Check sheet for the modelled part. Datum: model origin and axes. Units: mm. Coordinates: 2 decimals unless noted, no trailing zeros. Order: outer loops, then holes, each group sorted by start corner. A loop starts at its lowest first (then second) coordinate and runs counter-clockwise, first axis right, second up.
1. Thickness scan on line 1 (Y direction, x = 0.5, z = -2); line 2 (Y direction, x = 0.9, z = 1); line 3 (X direction, y = 12, z = -0.5). Record the ranges inside material, lowest first.
2. Cross-section at A-A (x = 0). Enter the section's corners in (y, z) (3 decimals).
3. Cross-section at C-C (y = 10.5). Enter the section's corners in (x, z).
4. Cross-section at B-B (z = 0). Enter the section's corners in (x, y), then the cut area to 3 significant figures.
```python
from build123d import *

# Parameters (mm, degrees)
SCHIZZO2_W                   = 5
SCHIZZO2_H                   = 8.75
ESTRUSIONE_ESTRUSIONE1_DEPTH = 120


with BuildPart() as part:
    # Schizzo1 → Rivoluzione2 (revolve)
    with BuildSketch(Plane.XY):
        with BuildLine():
            Line((-1.5, 0), (-1.5, 28.5))
            ThreePointArc((-1.5, 28.5), (-1.060660172, 29.560660172), (0, 30))
            Line((0, 30), (0, 0))
            Line((0, 0), (-1.5, 0))
        make_face()
    revolve(axis=Axis((0, 0, 0), (0, 1, 0)))

    # Schizzo2 → Estrusione-Estrusione1 (add)
    with BuildSketch(Plane.XZ):
        Rectangle(SCHIZZO2_W, SCHIZZO2_H)
    extrude(amount=ESTRUSIONE_ESTRUSIONE1_DEPTH)


solid = part.part
```
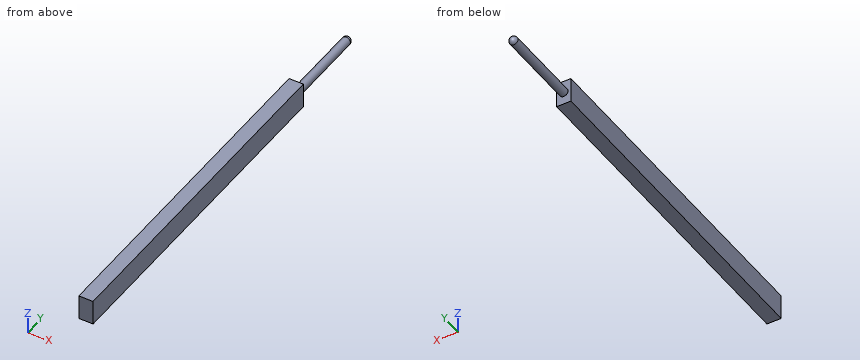
Data:
1. line 1: y = -120 to 0
1. line 2: y = -120 to 29.16
1. line 3: x = -1.41 to 1.41
2. outline: (-120, -4.375) - (0, -4.375) - (0, -1.5) - (28.5, -1.5) arc R1.5 ccw to (28.5, 1.5) - (0, 1.5) - (0, 4.375) - (-120, 4.375) - close
3. outline: circle Ø3 at (0, 0)
4. outline: (-2.5, -120) - (2.5, -120) - (2.5, 0) - (1.5, 0) - (1.5, 28.5) arc R1.5 ccw to (-1.5, 28.5) - (-1.5, 0) - (-2.5, 0) - close
4. area: 689 mm2
